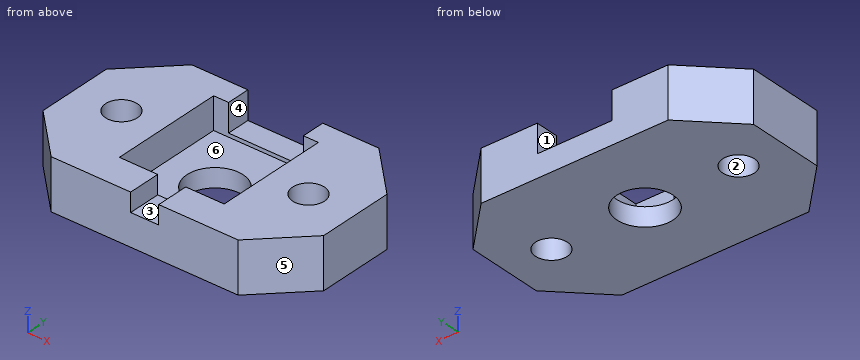
Autodesk Inventor part; units mm, degrees
ref_plane "YZ Plane" through (0, 0, 0) normal (1, 0, 0) x (0, 1, 0)
ref_plane "XZ Plane" through (0, 0, 0) normal (0, 1, 0) x (-1, 0, 0)
ref_plane "XY Plane" through (0, 0, 0) normal (0, 0, 1) x (1, 0, 0)
sketch "スケッチ1" plane through (0, 0, 0) normal (0, 0, 1) x (1, 0, 0)
  line L0 (0, 0) -> (11.2, 0)
  line L1 (11.2, 0) -> (11.2, 12.2)
  line L2 (11.2, 12.2) -> (0, 12.2)
  line L3 (0, 12.2) -> (0, 0)
  line L4 (-9.4, -3.5) -> (20.6, -3.5)
  line L5 (20.6, -3.5) -> (20.6, 14.7)
  line L6 (20.6, 14.7) -> (-9.4, 14.7)
  line L7 (-9.4, 14.7) -> (-9.4, -3.5)
  dimension "d0" = 11.2
  dimension "d1" = 12.2
  dimension "d2" = 2.5
  dimension "d3" = 3.5
  dimension "d4" = 9.4
  dimension "d5" = 9.4
extrude "押し出し1" add sketch "スケッチ1" along normal blind 3.4
extrude "押し出し2" add sketch "スケッチ1" against normal blind 2 contours L3 L2 L1 L0 | L7 L6 L5 L4
sketch "スケッチ2" plane through (0, 0, 3.4) normal (0, 0, 1) x (1, 0, 0)
  line L0 (11.2, 0) -> (0, 0)
  line L1 (0, 12.2) -> (11.2, 12.2)
  point P0 (5.6, 5.6)
  dimension "d41" = 6.6
hole "穴1" at (5.6, 5.6, 3.4) direction (0, 0, -1) diameter 6 end through all
sketch "スケッチ3" plane through (0, 0, 3.4) normal (0, 0, 1) x (1, 0, 0)
  line L0 (0, 12.2) -> (11.2, 12.2)
  line L1 (-9.4, 14.7) -> (20.6, 14.7)
  line L2 (9.6, 12.2) -> (1.6, 12.2)
  line L3 (1.6, 12.2) -> (1.6, 14.7)
  line L4 (1.6, 14.7) -> (9.6, 14.7)
  line L5 (9.6, 14.7) -> (9.6, 12.2)
  line L6 (-9.4, 14.7) -> (-9.4, -3.5)
  line L7 (20.6, -3.5) -> (20.6, 14.7)
  point P0 (0, 0)
  point P1 (9.6, 14.7)
  dimension "d17" = 8
  dimension "d18" = 11
  dimension "d33" = 30
extrude "押し出し3" cut sketch "スケッチ3" against normal blind 3
sketch "スケッチ4" plane through (0, 0, -2) normal (0, 0, -1) x (-1, 0, 0)
  circle A0 centre (-5.6, 5.6) radius 3
  line L0 (-20.6, -3.5) -> (9.4, -3.5)
  line L1 (9.4, 14.7) -> (-20.6, 14.7)
  point P0 (0, 0)
  point P1 (-15.6, 5.6)
  point P2 (4.4, 5.6)
  dimension "d21" = 20
  dimension "d22" = 10
  dimension "d23" = 10
  dimension "d24" = 9.1
  dimension "d25" = 18.2
hole "穴2" at (15.6, 5.6, -2) at (-4.4, 5.6, -2) direction (0, 0, 1) diameter 3.4 end through all
sketch "スケッチ5" plane through (0, 0, 3.4) normal (0, 0, 1) x (1, 0, 0)
  line L0 (20.6, -3.5) -> (-9.4, -3.5)
  line L1 (11.2, 0) -> (0, 0)
  line L2 (7.1, -3.5) -> (4.1, -3.5)
  line L3 (4.1, -3.5) -> (4.1, 0)
  line L4 (4.1, 0) -> (7.1, 0)
  line L5 (7.1, 0) -> (7.1, -3.5)
  line L6 (-9.4, 14.7) -> (-9.4, -3.5)
  point P0 (7.1, 0)
  dimension "d34" = 3
  dimension "d35" = 13.5
extrude "押し出し4" cut sketch "スケッチ5" against normal blind 2
chamfer "面取り1" distance 5 angle 45 4 edges at (20.6, -3.5, 0.7) (20.6, 14.7, 0.7) (-9.4, -3.5, 0.7) (-9.4, 14.7, 0.7)
properties part number "_3D プリント"
Could you check a few things on this model? Use its own coordinates, in mm. Face numbers are marked on the shaded views. A direction names the side the tool comes from. Give positions to 0.01 mm unless a question says otherwise; leave off trailing zeros. Loops run counter-clockwise (first coordinate to the right, second up) from the corner with the lowest first, then second, coordinate; pieces in that order, holes last. Notation, with made-up numbers: (27, 4) - (60, 4) arc R8 ccw to (60, 8) - close; hole circle Ø6 at (-29, -17). An arc over 180 degrees is marked (long way). Use one line per item in the form item = value.
1. I need wall thicknesses on probe 1 along X at (y, z) = (5.6, -0.8); probe 2 along X at (y, z) = (5.6, 1.4); probe 3 along Y at (x, z) = (-4.4, 1.45). Which ranges of each line are inside material? Lowest first, please.
Response values:
probe_1 = -9.4 to -6.1, -2.7 to 2.6, 8.6 to 13.9, 17.3 to 20.6
probe_2 = -9.4 to -6.1, -2.7 to 0, 11.2 to 13.9, 17.3 to 20.6
probe_3 = -3.5 to 3.9, 7.3 to 14.7
2. I want a section at A-A (x = 5.6). Please give me the cut outline in (y, z).
Response values:
outline = (-3.5, -2) - (2.6, -2) - (2.6, 0) - (0, 0) - (0, 1.4) - (-3.5, 1.4) - close; (8.6, -2) - (14.7, -2) - (14.7, 0.4) - (12.2, 0.4) - (12.2, 0) - (8.6, 0) - close
3. I want a section at D-D (x = 10). Please give me the cut outline in (y, z).
Response values:
outline = (-3.5, -2) - (14.7, -2) - (14.7, 3.4) - (12.2, 3.4) - (12.2, 0) - (0, 0) - (0, 3.4) - (-3.5, 3.4) - close
4. Thinking about a two-plate mould opening in Y: for the marked faces 4, 5 and 6, which applies, released by +Y, released by -Y, zero draft, split by the parting line, or undercut?
Response values:
face_4 = zero draft
face_5 = released by -Y
face_6 = undercut
5. I'm going to push flat-ended pins straight in: pin 1 Ø2 at (x, y) = (4, 14) entering from +Z; pin 2 Ø3 at (y, z) = (13.5, 2.5) entering from -X; pin 3 Ø5 at (x, y) = (5.6, 5.6) entering from +Z; pin 4 Ø5.5 at (x, y) = (6, 7.5) entering from +Z. Where does each tip first touch, or does it pass through?
Response values:
pin_1 = 0.4
pin_2 = -7.1
pin_3 = through
pin_4 = 0
6. I want a section at B-B (z = 2.4). Please give me the cut outline in (x, y).
Response values:
outline = (-9.4, 1.5) - (-4.4, -3.5) - (4.1, -3.5) - (4.1, 0) - (0, 0) - (0, 12.2) - (1.6, 12.2) - (1.6, 14.7) - (-4.4, 14.7) - (-9.4, 9.7) - close; (7.1, -3.5) - (15.6, -3.5) - (20.6, 1.5) - (20.6, 9.7) - (15.6, 14.7) - (9.6, 14.7) - (9.6, 12.2) - (11.2, 12.2) - (11.2, 0) - (7.1, 0) - close; hole circle Ø3.4 at (-4.4, 5.6); hole circle Ø3.4 at (15.6, 5.6)
7. I want a section at C-C (y = 5.6). Please give me the cut outline in (x, z), and give its area (3 significant figures).
Response values:
outline = (-9.4, -2) - (-6.1, -2) - (-6.1, 3.4) - (-9.4, 3.4) - close; (-2.7, -2) - (2.6, -2) - (2.6, 0) - (0, 0) - (0, 3.4) - (-2.7, 3.4) - close; (8.6, -2) - (13.9, -2) - (13.9, 3.4) - (11.2, 3.4) - (11.2, 0) - (8.6, 0) - close; (17.3, -2) - (20.6, -2) - (20.6, 3.4) - (17.3, 3.4) - close
area = 75.2 mm²
8. On a 3-axis mill with a long thin cutter (end or side, diameter ignored), from which of +Z, -Z, +X, -X, +Y, -Y can I reach the whole of each face in a straight line? I mean the marked faces 1, 2 and 3. Say none if no direction works.
Response values:
face_1 = +Z, +Y
face_2 = +Z, -Z
face_3 = +Z, +Y, -Y
